Read the model definition and answer for the solid it produces. Units are mm, in the model's axes. Face numbers are marked on the shaded views. A direction names the side the tool comes from. Give positions to 0.01 mm unless a question says otherwise; leave off trailing zeros. Loops run counter-clockwise (first coordinate to the right, second up) from the corner with the lowest first, then second, coordinate; pieces in that order, holes last.
(1) Straight lines are drawn through the part: probe 1 along Y at (x, z) = (14.25, 3.7); probe 2 along Y at (x, z) = (6.75, 3.5); probe 3 along Z at (x, y) = (-4.55, -35.9). For each, find the intervals that lie inside material, in ascending order.
(2) Find section A-A, the plane y = -35.9. Write down the section's boundary in (x, z).
(3) Each of these flat-tipped pins is pushed along its axis until it touches: P1, Ø1.5, axis at x = 14.25, y = -44, coming from the +Z side; P2, Ø1.6, axis at x = 9, y = 2, coming from the +Z side; P3, Ø14.5, axis at y = -36.5, z = 42, coming from the +X side. Where does it stop, or does it pass through?
(4) Find section D-D, the plane z = 17. Write down the section's boundary in (x, y), then the cut area to 3 significant figures.
(5) Which of the six approach directions +Z, -Z, +X, -X, +Y, -Y give full straight-line access (tool end or side, diameter ignored) to the marked faces 1, 2, 3 and 4?
(6) Determine the mould class of the marked faces 5, 6 and 7 for opening direction Y: pulls with the +Y half, pulls with the -Y half, needs draft (parallel to the pull), parting line crosses it, or undercut.
(7) Find section B-B, the plane z = 38. Write down the section's boundary in (x, y), then the cut area to 3 significant figures.
(8) Find section C-C, the plane x = 4.75. Write down the section's boundary in (y, z), then the cut area to 3 significant figures.
```python
from build123d import *

# Parameters (mm, degrees)
SKETCH_1_W          = 29
SKETCH_1_H          = 54
SKETCH_1_R          = 1.25
SKETCH_1_W_2        = 19
SKETCH_1_H_2        = 40
EXTRUDE_1_DEPTH     = 6
SKETCH_2_W          = 1.5
SKETCH_2_H          = 7
CUT_EXTRUDE_1_DEPTH = 2
SKETCH_3_R          = 8.1
EXTRUDE_2_DEPTH     = 5
SKETCH_4_R          = 9.1
CUT_EXTRUDE_2_DEPTH = 1
SKETCH_5_W          = 20
SKETCH_5_H          = 41
CUT_EXTRUDE_3_DEPTH = 71.072890621
SKETCH_6_R          = 6.5
CUT_EXTRUDE_4_DEPTH = 5


with BuildPart() as part:
    # Эскиз1 → Бобышка-Вытянуть1 (new body)
    with BuildSketch(Plane.XY):
        with Locations((9.5, -20)):
            Rectangle(SKETCH_1_W, SKETCH_1_H)
        with Locations((4.75, 4)):
            Circle(SKETCH_1_R, mode=Mode.SUBTRACT)
        with Locations((14.25, 4)):
            Circle(SKETCH_1_R, mode=Mode.SUBTRACT)
        with Locations((4.75, -44)):
            Circle(SKETCH_1_R, mode=Mode.SUBTRACT)
        with Locations((14.25, -44)):
            Circle(SKETCH_1_R, mode=Mode.SUBTRACT)
        with Locations((9.5, -20)):
            Rectangle(SKETCH_1_W_2, SKETCH_1_H_2, mode=Mode.SUBTRACT)
    extrude(amount=EXTRUDE_1_DEPTH)

    # Эскиз2 → Вырез-Вытянуть1 (cut)
    with BuildSketch(Plane.XY.offset(6)):
        with Locations((9.5, -43.5)):
            Rectangle(SKETCH_2_W, SKETCH_2_H)
        with Locations((9.5, 3.5)):
            Rectangle(SKETCH_2_W, SKETCH_2_H)
    extrude(amount=-CUT_EXTRUDE_1_DEPTH, mode=Mode.SUBTRACT)

    # Эскиз3 → Бобышка-Вытянуть2 (add)
    with BuildSketch(Plane(origin=(24, 0, 0), x_dir=(0, 0, -1), z_dir=(1, 0, 0))):
        with BuildLine():
            Line((-6, -47), (-41, -47))
            ThreePointArc((-41, -47), (-51.456010485, -39.625834772), (-48.019345484, -27.301233288))
            Line((-48.019345484, -27.301233288), (-6, 7))
            Line((-6, 7), (-6, -47))
        make_face()
        with Locations(Location((-41, -35.9, 0), (0, 0, 90))):
            Circle(SKETCH_3_R, mode=Mode.SUBTRACT)
    extrude_2 = extrude(amount=-EXTRUDE_2_DEPTH)

    # Эскиз4 → Вырез-Вытянуть2 (cut)
    with BuildSketch(Plane(origin=(24, 0, 0), x_dir=(0, 0, -1), z_dir=(1, 0, 0))):
        with Locations(Location((-41, -35.9, 0), (0, 0, 90))):
            Circle(SKETCH_4_R)
    cut_extrude_2 = extrude(amount=-CUT_EXTRUDE_2_DEPTH, mode=Mode.SUBTRACT)

    # Зеркальное отражение1: Бобышка-Вытянуть2, Вырез-Вытянуть2 across plane
    add(extrude_2.mirror(Plane.ZY.offset(-9.5)))
    add(cut_extrude_2.mirror(Plane.ZY.offset(-9.5)), mode=Mode.SUBTRACT)

    # Эскиз5 → Вырез-Вытянуть3 (cut, through all)
    with BuildSketch(Plane.XY.offset(6)):
        with Locations((9.5, -20)):
            Rectangle(SKETCH_5_W, SKETCH_5_H)
    extrude(amount=CUT_EXTRUDE_3_DEPTH, mode=Mode.SUBTRACT)

    # Эскиз6 → Вырез-Вытянуть4 (cut)
    with BuildSketch(Plane(origin=(24, 0, 0), x_dir=(0, 0, -1), z_dir=(1, 0, 0))):
        with Locations(Location((-21.633408306, -20.090663323, 0), (0, 0, 90))):
            Circle(SKETCH_6_R)
    extrude(amount=-CUT_EXTRUDE_4_DEPTH, mode=Mode.SUBTRACT)


solid = part.part
```
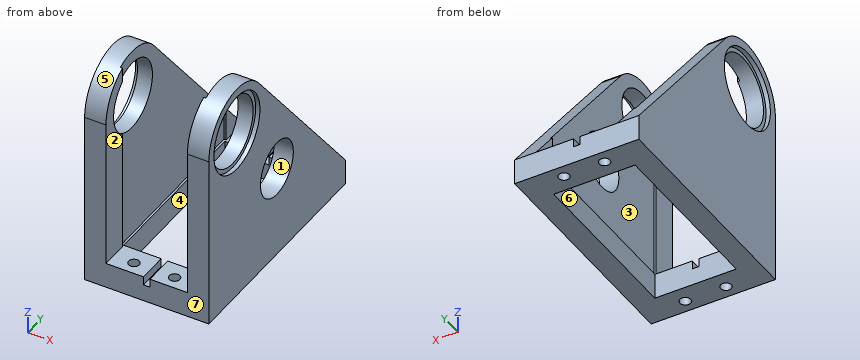
Entries:
1. probe 1: y = -47 to -45.25, -42.75 to -40, 0 to 2.75, 5.25 to 7
1. probe 2: y = -47 to -40, 0 to 7
1. probe 3: z = 0 to 31.9, 50.1 to 52.1
2. outline: (-5, 0) - (0, 0) - (0, 6) - (-0.5, 6) - (-0.5, 32.9) - (-4, 32.9) - (-4, 31.9) - (-5, 31.9) - close; (-5, 50.1) - (-4, 50.1) - (-4, 49.1) - (-0.5, 49.1) - (-0.5, 52.1) - (-5, 52.1) - close; (19, 0) - (24, 0) - (24, 31.9) - (23, 31.9) - (23, 32.9) - (19.5, 32.9) - (19.5, 6) - (19, 6) - close; (19.5, 49.1) - (23, 49.1) - (23, 50.1) - (24, 50.1) - (24, 52.1) - (19.5, 52.1) - close
3. P1: passes through
3. P2: stops at z = 6
3. P3: stops at x = 23
4. outline: (-5, -47) - (0, -47) - (0, -40.5) - (-0.5, -40.5) - (-0.5, -1.98) - (-5, -1.98) - close; (19, -47) - (24, -47) - (24, -24.65) - (19.5, -24.65) - (19.5, -40.5) - (19, -40.5) - close; (19.5, -15.53) - (24, -15.53) - (24, -1.98) - (19.5, -1.98) - close
4. area: 371 mm2
5. face 1: +X
5. face 2: +Z, +Y, -Y
5. face 3: +Z
5. face 4: +Z, -Z
6. face 5: parting line crosses it
6. face 6: undercut
6. face 7: pulls with the -Y half
7. outline: (-5, -47) - (0, -47) - (0, -43.42) - (-4, -43.42) - (-4, -44.49) - (-5, -44.49) - close; (-5, -27.31) - (-4, -27.31) - (-4, -28.38) - (-0.5, -28.38) - (-0.5, -19.12) - (-5, -19.12) - close; (19, -47) - (24, -47) - (24, -44.49) - (23, -44.49) - (23, -43.42) - (19, -43.42) - close; (19.5, -28.38) - (23, -28.38) - (23, -27.31) - (24, -27.31) - (24, -19.12) - (19.5, -19.12) - close
7. area: 115 mm2
8. outline: (-47, 0) - (-45.25, 0) - (-45.25, 6) - (-47, 6) - close; (-42.75, 0) - (-40, 0) - (-40, 6) - (-42.75, 6) - close; (0, 0) - (2.75, 0) - (2.75, 6) - (0, 6) - close; (5.25, 0) - (7, 0) - (7, 6) - (5.25, 6) - close
8. area: 54.0 mm2
